Part model, mm, in its own coordinate system. Face numbers are marked on the shaded views. A direction names the side the tool comes from. Coordinates: 2 decimals unless noted, no trailing zeros. Order: outer loops, then holes, each group sorted by start corner. A loop starts at its lowest first (then second) coordinate and runs counter-clockwise, first axis right, second up.
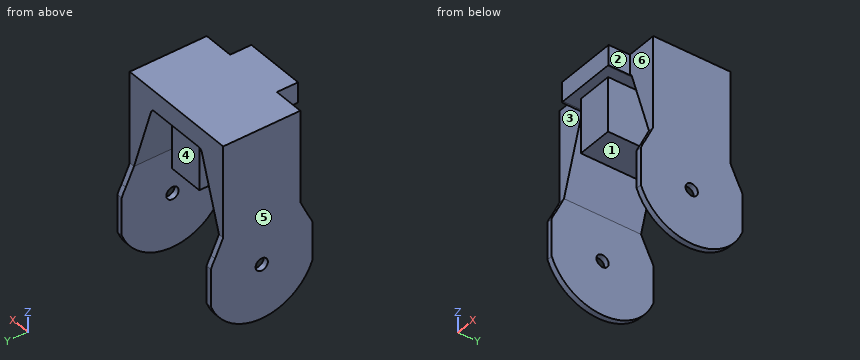
Autodesk Inventor part; units mm, degrees
ref_plane "Work Plane2" through (-27.5, 22, 41) normal (0, 1, 0) x (1, 0, 0)
ref_plane "Work Plane4" through (-27.5, 22, 41) normal (0, 0, 1) x (1, 0, 0)
ref_plane "Work Plane6" through (0, -22, 32) normal (1, 0, 0) x (0, 1, 0)
sketch "Sketch1" plane through (0, 0, 0) normal (0, 0, 1) x (1, 0, 0)
  line L0 (-27.5, 22) -> (27.5, 22)
  line L1 (27.5, 22) -> (27.5, -22)
  line L2 (27.5, -22) -> (-27.5, -22)
  line L3 (-27.5, -22) -> (-27.5, 22)
  line L4 (-27.5, 22) -> (27.5, -22) construction
  line L5 (27.5, 22) -> (-27.5, -22) construction
  point P0 (0, 0)
  dimension "d0" = 55
  dimension "d1" = 44
extrude "Extrusion1" add sketch "Sketch1" along normal blind 41
ref_plane "Work Plane2" through (-27.5, 22, 41) normal (0, 1, 0) x (1, 0, 0)
sketch "Sketch4" plane through (-27.5, 22, 41) normal (0, 1, 0) x (1, 0, 0)
  line L0 (42, 9) -> (13, 9)
  line L1 (2.5, 41) -> (13, 9)
  line L2 (42, 9) -> (52.5, 41)
  line L3 (2.5, 41) -> (52.5, 41)
  point P0 (27.5, 41)
  point P1 (55, 41)
extrude "Extrusion2" cut sketch "Sketch4" against normal blind 44
ref_plane "Work Plane4" through (-27.5, 22, 41) normal (0, 0, 1) x (1, 0, 0)
sketch "Sketch6" plane through (-27.5, 22, 41) normal (0, 0, 1) x (1, 0, 0)
  line L0 (0, 0) -> (0, -44)
  line L1 (0, -44) -> (0, -34.5)
  line L2 (55, -34.5) -> (55, -44)
  line L3 (13.75, -44) -> (13.75, -34.5)
  line L4 (41.25, -44) -> (41.25, -34.5)
  line L5 (0, -34.5) -> (13.75, -34.5)
  line L6 (41.25, -34.5) -> (55, -34.5)
  line L7 (55, -44) -> (41.25, -44)
  line L8 (13.75, -44) -> (0, -44)
  point P0 (27.5, -22)
extrude "Extrusion3" cut sketch "Sketch6" against normal blind 44
fillet "Fillet1" radius 2 1 edges at (14.5, 4.75, 32)
fillet "Fillet2" radius 2 1 edges at (-14.5, 4.75, 32)
sketch "Sketch7" plane through (27.5, 22, 41) normal (1, 0, 0) x (0, 0, -1)
  line L0 (41, 0) -> (41, -34.5)
  line L1 (61, 5.5) -> (52.6036, 5.5)
  line L2 (61, 5.5) -> (69.3964, 5.5)
  line L3 (61, -40) -> (52.6036, -40)
  line L4 (61, -40) -> (69.3964, -40)
  circle A0 centre (61, -17.25) radius 2.75
  line L5 (48.7056, 3.6524) -> (41, 0)
  line L6 (41, -34.5) -> (48.7056, -38.1524)
  arc A1 (69.3964, -40) -> (69.3964, 5.5) centre (61, -17.25) ccw
  arc A2 (52.6036, 5.5) -> (48.7056, 3.6524) centre (61, -17.25) ccw
  arc A3 (48.7056, -38.1524) -> (52.6036, -40) centre (61, -17.25) ccw
  line L7 (41, 0) -> (41, -34.5)
  point P0 (0, -22)
  dimension "d25" = 5.5
ref_plane "Work Plane6" through (0, -22, 32) normal (1, 0, 0) x (0, 1, 0)
extrude "Extrusion4" add sketch "Sketch7" against normal blind 2.5
mirror "Mirror1" about plane through (0, -22, 32) normal (1, 0, 0) of "Extrusion4"
sketch "Sketch14" plane through (0, -22, 32) normal (1, 0, 0) x (0, 1, 0)
  point P0 (22, -32)
ref_plane "Work Plane11" through (-13.0513, -22, 32) normal (0, 0, -1) x (-1, 0, 0)
sketch "Sketch15" plane through (-13.0513, -22, 32) normal (0, 0, -1) x (-1, 0, 0)
  line L0 (-21.0513, 39.8663) -> (-5.0513, 39.8663)
  line L1 (-5.0513, 39.8663) -> (-5.0513, 4.1337)
  line L2 (-5.0513, 4.1337) -> (-21.0513, 4.1337)
  line L3 (-21.0513, 4.1337) -> (-21.0513, 39.8663)
  line L4 (-21.0513, 39.8663) -> (-5.0513, 4.1337) construction
  line L5 (-5.0513, 39.8663) -> (-21.0513, 4.1337) construction
  point P0 (-13.0513, 22)
  dimension "d49" = 16
extrude "Extrusion8" add sketch "Sketch15" along normal blind 24.5
sketch "Sketch10" plane through (27.5, 22, 41) normal (0, 0, 1) x (1, 0, 0)
  line L0 (-52, -17.25) -> (-52, -10.25)
  line L1 (-52, -17.25) -> (-52, -24.25)
  line L2 (-52, -10.25) -> (-47.299, -10.25)
  line L3 (-52, -24.25) -> (-47.299, -24.25)
  line L4 (-3, -17.25) -> (-3, -10.25)
  line L5 (-3, -17.25) -> (-3, -24.25)
  line L6 (-3, -10.25) -> (-7.701, -10.25)
  line L7 (-3, -24.25) -> (-7.701, -24.25)
  arc A0 (-47.299, -24.25) -> (-7.701, -24.25) centre (-27.5, -17.25) ccw
  arc A1 (-7.701, -10.25) -> (-47.299, -10.25) centre (-27.5, -17.25) ccw
  circle A2 centre (-27.5, -17.25) radius 2.75
  point P0 (-27.5, -22)
  point P1 (-55, 0)
  dimension "d35" = 5.5
sketch "Sketch11" plane through (-24.5, 11.75, 43.5) normal (0, 0, 1) x (1, 0, 0)
  line L0 (0, 0) -> (49, 0)
  line L1 (49, 0) -> (49, -5)
  line L2 (49, -5) -> (0, -5)
  line L3 (0, -5) -> (0, 0)
  point P0 (24.5, -11.75)
  dimension "d39" = 5
sketch "Sketch13" plane through (-24.5, 6.75, 81.5) normal (0, -1, 0) x (1, 0, 0)
  line L0 (49, 0) -> (64, 0)
  line L1 (49, -38) -> (26.3875, -38)
  line L2 (49, 0) -> (49, -38)
  line L3 (64, 0) -> (49, -38)
  line L4 (0, -40.5) -> (0, 0)
  line L5 (0, 0) -> (-15, 0)
  line L6 (0, -38) -> (4.701, -38)
  line L7 (-15, 0) -> (0, -38)
  line L8 (0, -38) -> (0, 0)
  point P0 (24.5, -81.5)
  dimension "d45" = 15
  dimension "d46" = 15
properties part number "hand"
(1) Slice it at C-C, the plane z = 6. Give the cut face in (x, y), then the cut area to 3 significant figures.
(2) Slice it at B-B, the plane y = 4.75. Give the cut face in (x, z), then the cut area to 3 significant figures.
(3) Probe line 1 (X direction, y = 5.5, z = -27.5); line 2 (Y direction, x = 26, z = -20); line 3 (X direction, y = -4.5, z = 9.5). List the from-to ranges inside material, lowest first.
(4) Slice it at D-D, the plane x = -9.5. Give the cut face in (y, z), then the cut area to 3 significant figures.
(5) Pull direction X, two halves, no side cores. Call the marked faces 4, 5 and 6: +X half, -X half, draft (parallel to the pull), parting line (faces both ways), or undercut.
(6) Drop flat-ended pins along their axis: pin 1 (8 mm diameter, centred on x = 2.5, z = 18.5, fed in from -Y); pin 2 (1.2 mm diameter, centred on x = 26.5, z = -19, fed in from -Y); pin 3 (2 mm diameter, centred on x = -11.5, y = 1.5, fed in from -Z); pin 4 (7.5 mm diameter, centred on y = -15.5, z = 36, fed in from -X). Give the stop position or say it passes through.
(7) Slice it at A-A, the plane z = -20. Give the cut face in (x, y), then the cut area to 3 significant figures.
(8) Tool access for the marked faces 1, 2 and 3: list every direction of +Z, -Z, +X, -X, +Y, -Y with a clear straight run to the whole face (end or side of a thin tool).
Here are the results:
1. outline: (-27.5, -12.5) - (-23.03, -12.5) - (-23.03, 22) - (-27.5, 22) - close; (23.03, -12.5) - (27.5, -12.5) - (27.5, 22) - (23.03, 22) - close
1. area: 308 mm2
2. outline: (-27.5, -44.25) - (-25, -44.25) - (-25, -22.75) - (-27.5, -22.75) - close; (-27.5, -17.25) - (-25, -17.25) - (-25, 0) - (-14.95, 30.62) arc R2 cw to (-13.05, 32) - (-8, 32) - (-8, 7.5) - (8, 7.5) - (8, 32) - (13.05, 32) arc R2 cw to (14.95, 30.62) - (25, 0) - (25, -17.25) - (27.5, -17.25) - (27.5, 41) - (-27.5, 41) - close; (25, -44.25) - (27.5, -44.25) - (27.5, -22.75) - (25, -22.75) - close
2. area: 1,580 mm2
3. line 1: x = -27.5 to -25, 25 to 27.5
3. line 2: y = -18 to 2, 7.5 to 27.5
3. line 3: x = -27.5 to -21.88, -8 to 8, 21.88 to 27.5
4. outline: (-22, 32) - (22, 32) - (22, 41) - (-22, 41) - close
4. area: 396 mm2
5. face 4: undercut
5. face 5: -X half
5. face 6: draft
6. pin 1: stops at y = -17.87
6. pin 2: stops at y = -18
6. pin 3: stops at z = 32
6. pin 4: stops at x = -27.5
7. outline: (-27.5, -18) - (-25, -18) - (-25, 2) - (-27.5, 2) - close; (-27.5, 7.5) - (-25, 7.5) - (-25, 27.5) - (-27.5, 27.5) - close; (25, -18) - (27.5, -18) - (27.5, 2) - (25, 2) - close; (25, 7.5) - (27.5, 7.5) - (27.5, 27.5) - (25, 27.5) - close
7. area: 200 mm2
8. face 1: -Z, +Y, -Y
8. face 2: +Z, -Z, +X, -Y
8. face 3: +Z, -X, -Y
